Read the model definition and answer for the solid it produces. Units are mm, in the model's axes. Face numbers are marked on the shaded views. A direction names the side the tool comes from. Coordinates: 2 decimals unless noted, no trailing zeros. Loops run counter-clockwise (first coordinate to the right, second up) from the corner with the lowest first, then second, coordinate; pieces in that order, holes last.
from build123d import *

# Parameters (mm, degrees)
F0_R           = 8.7249
F1_DEPTH       = 25.4
F2_R           = 9.525
F3_DEPTH       = 50.8
F4_W           = 6.604
F4_H           = 31.75
F4_W_2         = 7.7840778498
F4_H_2         = 37.4901928008
F5_DEPTH       = 25.4
F5_DEPTH_BACK  = 25.4
F6_R           = 2.54
F7_SIZE        = 0.508
F8_T4_DEPTH    = 22.6820176921
F8_S5_R        = 9.525
F8_T6_DEPTH    = 13
F8_T10_DEPTH   = 22.6820176921
F8_S11_R       = 9.525
F8_T12_DEPTH   = 13
F9_R           = 3.175
F10_DEPTH      = 25.4
F10_DEPTH_BACK = 25.4
F11_R          = 1.778
F12_R          = 6.35
F13_DEPTH      = 25.4


# Not quite as in the source:
# - a fillet or chamfer that OpenCascade refuses, or shapes differently, is made with other operations: its cross-section is extruded or revolved along the edge and cut away or added


with BuildPart() as f1:
    # F0 (on Top) → F1 (new body)
    with BuildSketch(Plane.XY):
        Circle(F0_R)
    extrude(amount=F1_DEPTH)

    # F2 (on face) → F3 (join)
    with BuildSketch(Plane.XY.offset(25.4)):
        Circle(F2_R)
    extrude(amount=F3_DEPTH)

    # F4 (on Front) → F5 (cut, two sides)
    with BuildSketch(Plane.XZ) as f5_sk:
        with Locations((0, 63.5)):
            Rectangle(F4_W, F4_H)
        with Locations((12.0047114623, 66.3700964004)):
            Rectangle(F4_W_2, F4_H_2)
        with Locations((-12.0047114623, 66.3700964004)):
            Rectangle(F4_W_2, F4_H_2)
    extrude(amount=-F5_DEPTH, mode=Mode.SUBTRACT)
    extrude(f5_sk.sketch, amount=F5_DEPTH_BACK, mode=Mode.SUBTRACT)

    # F6
    f6_edges = [f1.edges().sort_by_distance(p)[0] for p in [
        (-3.302, 0, 47.625),
        (3.302, 0, 47.625),
    ]]
    fillet(f6_edges, radius=F6_R)

    # F7
    f7_edges = [f1.edges().sort_by_distance(p)[0] for p in [
        (3.302, 0, 76.2),
        (-3.302, 0, 76.2),
        (-8.112673, 0, 76.2),
        (8.112673, 0, 76.2),
    ]]
    chamfer(f7_edges, length=F7_SIZE)

    # F8: fillet of radius 2.54 on 2 edges, made by hand


with BuildPart() as f8_tool2:
    # F8_s3 → F8_t4 (new body)
    with BuildSketch(Plane.XZ.offset(11.341008846)):
        with BuildLine():
            ThreePointArc((8.1126725374, 50.165), (8.8566213132, 48.3689487758), (10.6526725374, 47.625))
            Line((10.6526725374, 47.625), (8.1126725374, 47.625))
            Line((8.1126725374, 47.625), (8.1126725374, 50.165))
        make_face()
    extrude(amount=-F8_T4_DEPTH)

    # F8_s5 → F8_t6 (intersect, symmetric)
    with BuildSketch(Plane.XY.offset(48.9)):
        Circle(F8_S5_R)
    extrude(amount=F8_T6_DEPTH, both=True, mode=Mode.INTERSECT)


with BuildPart() as f1_1:
    add(f1.part)

    # F8_t1: union F8_tool2
    add(f8_tool2.part)


with BuildPart() as f8_tool8:
    # F8_s9 → F8_t10 (new body)
    with BuildSketch(Plane.XZ.offset(11.341008846)):
        with BuildLine():
            ThreePointArc((-8.1126725374, 50.165), (-8.8566213132, 48.3689487758), (-10.6526725374, 47.625))
            Line((-10.6526725374, 47.625), (-8.1126725374, 47.625))
            Line((-8.1126725374, 47.625), (-8.1126725374, 50.165))
        make_face()
    extrude(amount=-F8_T10_DEPTH)

    # F8_s11 → F8_t12 (intersect, symmetric)
    with BuildSketch(Plane.XY.offset(48.9)):
        Circle(F8_S11_R)
    extrude(amount=F8_T12_DEPTH, both=True, mode=Mode.INTERSECT)


with BuildPart() as f1_2:
    add(f1_1.part)

    # F8_t7: union F8_tool8
    add(f8_tool8.part)

    # F9 (on face) → F10 (cut, two sides)
    with BuildSketch(Plane(origin=(-8.1126725374, 0, 0), x_dir=(0, -1, 0), z_dir=(-1, 0, 0))) as f10_sk:
        with Locations((0, 69.85)):
            Circle(F9_R)
    extrude(amount=-F10_DEPTH, mode=Mode.SUBTRACT)
    extrude(f10_sk.sketch, amount=F10_DEPTH_BACK, mode=Mode.SUBTRACT)

    # F11
    f11_edges = [f1_2.edges().sort_by_distance(p)[0] for p in [
        (-5.900452, 7.477318, 76.2),
        (5.900452, 7.477318, 76.2),
    ]]
    fillet(f11_edges, radius=F11_R)

    # F12 (on face) → F13 (cut)
    with BuildSketch(Plane(origin=(0, 0, 0), x_dir=(1, 0, 0), z_dir=(0, 0, -1))):
        Circle(F12_R)
    extrude(amount=-F13_DEPTH, mode=Mode.SUBTRACT)


solid = f1_2.part
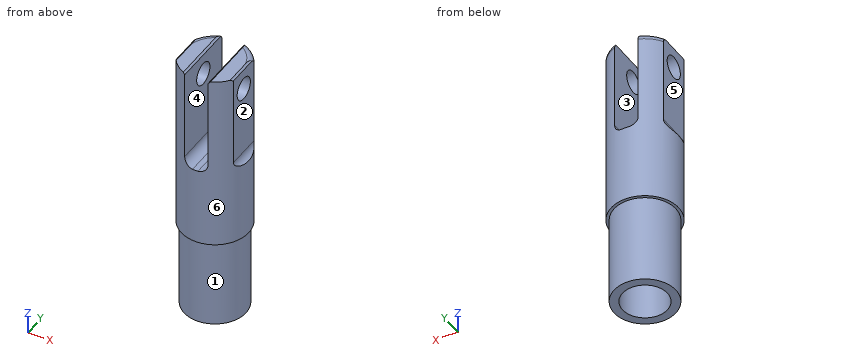
Q1. Flat-ended cylindrical pins translate along their axes: pin 1 Ø9 at (y, z) = (-1, 58.5) entering from -X; pin 2 Ø8 at (x, z) = (-0.5, 29.5) entering from +Y (3 decimals); pin 3 Ø5.5 at (y, z) = (-1, 69.5) entering from +X; pin 4 Ø1.5 at (x, y) = (3, -0.5) entering from -Z. Find the tip coordinate at first contact, or state that the pin passes through.
Findings below:
pin 1: stops at x = -8.11
pin 2: stops at y = 9.525
pin 3: stops at x = 8.11
pin 4: stops at z = 25.4
Q2. A cutting plane is placed at D-D (z = 22). Give the vertices of the cut face in (x, y), then the cut area to 3 significant figures.
Findings below:
outline: circle Ø17.45 at (0, 0); hole circle Ø12.7 at (0, 0)
area: 112 mm2
Q3. A cutting plane is placed at C-C (x = 0). Give the vertices of the cut face in (y, z) (3 decimals), then the cut area to 3 significant figures.
Findings below:
outline: (-9.525, 25.4) - (-8.725, 25.4) - (-8.725, 0) - (-6.35, 0) - (-6.35, 25.4) - (6.35, 25.4) - (6.35, 0) - (8.725, 0) - (8.725, 25.4) - (9.525, 25.4) - (9.525, 47.625) - (-9.525, 47.625) - close
area: 544 mm2
Q4. A cutting plane is placed at B-B (y = 0). Count the separate pieces of the cut face and the enclosed holes in it, then the cut area to 3 significant figures.
Findings below:
separate pieces: 3
enclosed holes: 0
area: 763 mm2
Q5. Straight lines are drawn through the part: probe 1 along Z at (x, y) = (-5.85, 0) (3 decimals); probe 2 along Y at (x, z) = (0.25, 10.5); probe 3 along X at (y, z) = (-1, 62). For each, find the intervals that lie inside material, in ascending order.
Findings below:
probe 1: z = 25.4 to 66.675, 73.025 to 76.2
probe 2: y = -8.72 to -6.35, 6.35 to 8.72
probe 3: x = -8.11 to -3.3, 3.3 to 8.11
Q6. A cutting plane is placed at A-A (z = 69.85). Give the vertices of the cut face in (x, y) (3 decimals), then the cut area to 3 significant figures.
Findings below:
outline: (-8.113, -4.991) arc R9.525 ccw to (-3.302, -8.934) - (-3.302, -3.175) - (-8.113, -3.175) - close; (-8.113, 3.175) - (-3.302, 3.175) - (-3.302, 8.934) arc R9.525 ccw to (-8.113, 4.991) - close; (3.302, -8.934) arc R9.525 ccw to (8.113, -4.991) - (8.113, -3.175) - (3.302, -3.175) - close; (3.302, 3.175) - (8.113, 3.175) - (8.113, 4.991) arc R9.525 ccw to (3.302, 8.934) - close
area: 81.6 mm2
Q7. Which of the six approach directions +Z, -Z, +X, -X, +Y, -Y give full straight-line access (tool end or side, diameter ignored) to the marked faces 1 and 2?
Findings below:
face 1: -Z
face 2: +Z, +X, +Y, -Y
Q8. Determine the mould class of the marked faces 3, 4, 5 and 6 for opening direction X: +X half, -X half, draft (parallel to the pull), parting line (faces both ways), or undercut.
Findings below:
face 3: undercut
face 4: undercut
face 5: -X half
face 6: parting line
